Solid Edge part; units mm, degrees
sketch "Sketch1" plane through (0, 0, 0) normal (0, 0, 1) x (1, 0, 0)
  circle A0 centre (0, 0) radius 27
extrude "Protrusion1" add sketch "Sketch1" along normal blind 45
hole "Agujero_1" at (0, 0, 45) direction (0, 0, -1) diameter 40 depth 5
hole "Agujero_3" at (0, 0, 40) direction (0, 0, -1) diameter 33 depth 26
fillet "Redondeo_1" radius 3 1 edges at (-27, 0, 0)
Work out the finished part from the listing and answer in its coordinate system (mm). A direction names the side the tool comes from. Give positions to 0.01 mm unless a question says otherwise; leave off trailing zeros. Loops run counter-clockwise (first coordinate to the right, second up) from the corner with the lowest first, then second, coordinate; pieces in that order, holes last. Notation, with made-up numbers: (83, 72) - (104, 72) arc R14 ccw to (104, 90) - close; hole circle Ø8 at (-25, -0.75). An arc over 180 degrees is marked (long way). Answer in a Markdown table with one row per item. Add a question column.
Q1. Each of these flat-tipped pins is pushed along its axis until it touches: P1, Ø1, axis at y = 6.5, z = 5, coming from the -X side; P2, Ø12, axis at x = 18.5, z = 13, coming from the +Y side; P3, Ø10, axis at y = -10.5, z = 19, coming from the -X side. Where does it stop, or does it pass through?
Q2. Determine the mould class of faces 3 (the cylindrical face through (-5.85, 26.36, 23.71)), 4 (the flat face through (0, 0, 0)), 5 (the cylindrical face through (6.32, -15.24, 26.82)) for opening direction X: released by +X, released by -X, zero draft, split by the parting line, or undercut.
Q3. Consider line 1 along Y through (x, z) = (0, 43.4); line 2 along Y through (x, z) = (0, 24); line 3 along X through (y, z) = (-4, 31.5). Determine where each line is inside the solid, lowest interval first.
Q4. The part is cut by section C-C (z = 15). Determine the outline of the cut face in (x, y).
Q5. The part is cut by section A-A (x = 0). Determine the outline of the cut face in (y, z).
Q6. A tool of negligible diameter and unlimited length cuts with its end or side. For faces 1 (the cylindrical face through (19.524, 4.336, 42.465)), 2 (the flat face through (-18, -10, 45)), from which of +Z, -Z, +X, -X, +Y, -Y can it reach the whole face along a straight path? Write none if from no direction.
Solution:
| question | item | result |
|---|---|---|
| 1 | P1 | stops at x = -26.32 |
| 1 | P2 | stops at y = 23.93 |
| 1 | P3 | stops at x = -26.43 |
| 2 | face 3 | split by the parting line |
| 2 | face 4 | zero draft |
| 2 | face 5 | undercut |
| 3 | line 1 | y = -27 to -20, 20 to 27 |
| 3 | line 2 | y = -27 to -16.5, 16.5 to 27 |
| 3 | line 3 | x = -26.7 to -16.01, 16.01 to 26.7 |
| 4 | outline | circle Ø54 at (0, 0); hole circle Ø33 at (0, 0) |
| 5 | outline | (-27, 3) arc R3 ccw to (-24, 0) - (24, 0) arc R3 ccw to (27, 3) - (27, 45) - (20, 45) - (20, 40) - (16.5, 40) - (16.5, 14) - (-16.5, 14) - (-16.5, 40) - (-20, 40) - (-20, 45) - (-27, 45) - close |
| 6 | face 1 | +Z |
| 6 | face 2 | +Z, +X, -X, +Y, -Y |
